Autodesk Inventor part; units mm, degrees
ref_plane "YZ Plane" through (0, 0, 0) normal (1, 0, 0) x (0, 1, 0)
ref_plane "XZ Plane" through (0, 0, 0) normal (0, 1, 0) x (-1, 0, 0)
ref_plane "XY Plane" through (0, 0, 0) normal (0, 0, 1) x (1, 0, 0)
sketch "Sketch1" plane through (0, 0, 0) normal (0, 1, 0) x (-1, 0, 0)
  circle A0 centre (0, 0) radius 57.5
  circle A1 centre (0, 0) radius 48
  circle A2 centre (0, 0) radius 50
  line L0 (0, 0) -> (7.5, 0)
  line L1 (7.5, 0) -> (-7.5, 0)
  line L2 (-7.5, 0) -> (-7.5, -47.4104)
  line L3 (7.5, 0) -> (7.5, -47.4104)
  line L4 (7.5, 0) -> (7.5, 47.4104)
  line L5 (-7.5, 0) -> (-7.5, 47.4104)
  dimension "d0" = 115
  dimension "d1" = 96
  dimension "d2" = 100
extrude "Extrusion1" add sketch "Sketch1" along normal blind 1 contours A0 | A1 L3 L4 | L4 L0 L1 L5 A1 | A1 L2 L1 L0 L3 | L5 L2 A1 | A2
sketch "Sketch2" plane through (0, 1, 0) normal (0, 1, 0) x (1, 0, 0)
  circle A0 centre (0, 0) radius 49
  circle A1 centre (0, 0) radius 50
  line L0 (0, 0) -> (7.5, 0)
  line L1 (7.5, -48.4226) -> (7.5, 48.4226)
  line L2 (7.5, 0) -> (7.5, 48.4226)
  line L3 (7.5, 48.4226) -> (7.5, -48.4226)
  line L4 (-7.5, 48.4226) -> (-7.5, -48.4226)
  dimension "d7" = 98
  dimension "d8" = 100
extrude "Extrusion2" add sketch "Sketch2" along normal blind 30 contours L1 A0 L4 | A1
sketch "Sketch3" plane through (0, 0, 0) normal (0, -1, 0) x (1, 0, 0)
  circle A0 centre (0, 0) radius 49
  line L0 (0, 0) -> (0, 40)
  line L1 (0, 40) -> (0, -40)
  dimension "d11" = 98
  dimension "d12" = 40
  dimension "d13" = 80
extrude "Extrusion3" cut sketch "Sketch3" against normal blind 30
sketch "Sketch4" plane through (0, 31, 0) normal (0, 1, 0) x (1, 0, 0)
  line L0 (0, 0) -> (0, -40)
  line L1 (0, -40) -> (-7.5, -40)
  line L2 (-7.5, 48.4226) -> (-7.5, -48.4226)
  line L3 (7.5742, -40) -> (0, -40)
  line L4 (7.5742, -40) -> (7.5, 40)
  line L5 (7.5, -48.4226) -> (7.5, 48.4226)
  line L6 (7.5, 40) -> (-7.5742, 39.986)
  line L7 (-7.5742, 39.986) -> (-7.5, -40)
  line L8 (-7.5, -40) -> (-7.5742, 39.986)
  line L9 (0, -40) -> (0, -42.5)
  line L10 (-0.0371, 39.993) -> (-0.0371, 42.493)
  circle A0 centre (-0.0371, 42.493) radius 1.025
  circle A1 centre (0, -42.5) radius 1.025
  point P0 (-7.5, 39.9861)
  point P1 (7.5, -40)
  dimension "d16" = 40
  dimension "d17" = 80
  dimension "d18" = 2.5
  dimension "d19" = 2.5
  dimension "d20" = 2.05
  dimension "d21" = 2.05
extrude "Extrusion4" cut sketch "Sketch4" against normal through all contours L1 L2 L6 L5 L3 | A0 | A1
sketch "Sketch5" plane through (0, 0, 0) normal (0, -1, 0) x (1, 0, 0)
  circle A0 centre (0, 0) radius 49
  circle A1 centre (0, 0) radius 48
  dimension "d24" = 98
  dimension "d25" = 96
extrude "Extrusion5" add sketch "Sketch5" against normal blind 31
sketch "Sketch6" plane through (0, 31, 0) normal (0, 1, 0) x (1, 0, 0)
  circle A0 centre (0, 0) radius 50
  circle A1 centre (0, -42.5) radius 1.025
  circle A2 centre (0, -42.5) radius 1.025
  line L0 (-7.5, -40) -> (-7.5, -47.4104)
  line L1 (-7.5, -47.4104) -> (-7.5, -40)
  line L2 (7.5, -47.4104) -> (7.5, -40)
  line L3 (-7.5, -40) -> (7.5, -40)
  line L4 (7.5, -40) -> (-7.5, -40)
  line L5 (-7.5, -47.4104) -> (-7.5, -40)
  line L6 (7.5, -40) -> (-7.5, -40)
  arc A3 (7.5, -47.4104) -> (7.5, 47.4104) centre (0, 0) ccw
  arc A4 (-7.5, 47.4104) -> (-7.5, -47.4104) centre (0, 0) ccw
  line L7 (7.5, 40) -> (7.5, 47.4104)
  line L8 (7.5, 47.4104) -> (7.5, 40)
  line L9 (7.5, 40) -> (-7.5, 40)
  line L10 (-7.5, 40) -> (-7.5, 47.4104)
  circle A5 centre (-0.0371, 42.493) radius 1.025
  circle A6 centre (-0.0371, 42.493) radius 1.025
  dimension "d28" = 100
  dimension "d30" = 2.05
  dimension "d31" = 2.05
extrude "Extrusion6" add sketch "Sketch6" along normal blind 4
properties part number "Chassis_Support"
Design review of the part built by this model. Coordinates are the model's own, in mm. A direction names the side the tool comes from. Round coordinates to 2 decimals unless told otherwise and drop trailing zeros. Loops run counter-clockwise (first coordinate to the right, second up) from the corner with the lowest first, then second, coordinate; pieces in that order, holes last. Notation, with made-up numbers: (-7, 45.25) - (31, 45.25) arc R24 cw to (31, 83.25) - close; hole circle Ø1 at (-11.75, 50.5). An arc over 180 degrees is marked (long way). One line per item, written item: value. Start each with the question number.
1) Consider section A-A on x = -38.5. Give the boundary of the cut face in (y, z), then the cut area to 3 significant figures.
2) For faces 4 (the flat face through (17.3, 1, 47.1)), 5 (the flat face through (-7.5, 32, -44)), 6 (the flat face through (0, 30, -44)), list the 3-axis set-ups (+Z, -Z, +X, -X, +Y, -Y) from which the entire face can be reached by the end or side of a thin tool; tool diameter is ignored.
3) Consider section C-C on y = 24.5. Give the boundary of the cut face in (x, z), then the cut area to 3 significant figures.
4) Consider section D-D on x = -12. Give the boundary of the cut face in (y, z), then the cut area to 3 significant figures.
5) Consider section B-B on z = -9. Give the boundary of the cut face in (x, y).
6) To check wall thickness, follow L1, parallel to Z at x = 0, y = 31.25 (3 decimals); L2, parallel to X at y = 13, z = 0; L3, parallel to X at y = 24.5, z = -31. State the ranges of each line that lie inside material, in increasing order. Write a range as from..to.
7) Draft analysis for pull direction X (two halves, no side actions). For faces 1 (the flat face through (0, 30, 44)), 2 (the cylindrical face through (47.69, 17.76, 15.02)), 3 (the flat face through (-13, 0, -47)), state which applies: +X half, -X half, draft (parallel to the pull), parting line (faces both ways), or undercut.
8) Insertion check: pin 1 Ø12 at (y, z) = (24.5, -41) entering from +X; pin 2 Ø1.5 at (x, z) = (28.5, -43.5) entering from +Y; pin 3 Ø10 at (y, z) = (27, 28.5) entering from +X. Each pin has a flat end and moves straight along its axis. Give the tip position at first contact, or say it passes through.
Reported:
1. outline: (0, -42.71) - (1, -42.71) - (1, -31.9) - (35, -31.9) - (35, -28.67) - (0, -28.67) - close; (0, 28.67) - (35, 28.67) - (35, 31.9) - (1, 31.9) - (1, 42.71) - (0, 42.71) - close
1. area: 248 mm^2
2. face 4: +Y
2. face 5: +Y, -Y
2. face 6: -Y
3. outline: circle Ø100 at (0, 0); hole circle Ø96 at (0, 0)
3. area: 616 mm^2
4. outline: (0, -56.23) - (1, -56.23) - (1, -48.54) - (35, -48.54) - (35, -46.48) - (0, -46.48) - close; (0, 46.48) - (35, 46.48) - (35, 48.54) - (1, 48.54) - (1, 56.23) - (0, 56.23) - close
4. area: 160 mm^2
5. outline: (-56.79, 0) - (-47.15, 0) - (-47.15, 35) - (-49.18, 35) - (-49.18, 1) - (-56.79, 1) - close; (47.15, 0) - (56.79, 0) - (56.79, 1) - (49.18, 1) - (49.18, 35) - (47.15, 35) - close
6. L1: z = -50..-43.517, -41.469..-40, 40..41.475, 43.525..50
6. L2: x = -50..-48, 48..50
6. L3: x = -39.23..-36.65, 36.65..39.23
7. face 1: undercut
7. face 2: parting line
7. face 3: draft
8. pin 1: stops at x = 35.71
8. pin 2: stops at y = 1
8. pin 3: stops at x = 44.13
